from build123d import *

# Parameters (mm, degrees)
F0_W     = 64
F0_H     = 150
F1_DEPTH = 1.5
F2_W     = 48
F2_H     = 39.9
F2_H_2   = 38.8
F2_H_3   = 39.3
F3_DEPTH = 1.501
F4_R     = 8
F6_DEPTH = 4


with BuildPart() as f1:
    # F0 (on Top) → F1 (new body)
    with BuildSketch(Plane.XY):
        with Locations((32, 75)):
            Rectangle(F0_W, F0_H)
    extrude(amount=F1_DEPTH)

    # F2 (on face) → F3 (cut, through all)
    with BuildSketch(Plane.XY.offset(1.5)):
        with Locations((32, 122.05)):
            Rectangle(F2_W, F2_H)
        with Locations((32, 74.7)):
            Rectangle(F2_W, F2_H_2)
        with Locations((32, 27.65)):
            Rectangle(F2_W, F2_H_3)
    extrude(amount=-F3_DEPTH, mode=Mode.SUBTRACT)

    # F4
    f4_edges = [f1.edges().sort_by_distance(p)[0] for p in [
        (8, 142, 0.75),
        (8, 94.1, 0.75),
        (8, 47.3, 0.75),
        (8, 102.1, 0.75),
        (8, 55.3, 0.75),
        (8, 8, 0.75),
        (56, 102.1, 0.75),
        (56, 55.3, 0.75),
        (56, 8, 0.75),
        (56, 142, 0.75),
        (56, 94.1, 0.75),
        (56, 47.3, 0.75),
    ]]
    fillet(f4_edges, radius=F4_R)

    # F5 (on face) → F6 (join)
    with BuildSketch(Plane.XY.offset(1.5)):
        Polygon((0, 0), (64, 0), (64, 0.5), (0.5, 0.5), (0.5, 149.5), (64, 149.5), (64, 150), (0, 150), align=None)
    extrude(amount=F6_DEPTH)


solid = f1.part
Geometry: final body of the model. Coordinates: model frame, mm. A direction names the side the tool comes from. Give positions to 0.01 mm unless a question says otherwise; leave off trailing zeros. Loops run counter-clockwise (first coordinate to the right, second up) from the corner with the lowest first, then second, coordinate; pieces in that order, holes last. Notation, with made-up numbers: (19, -4) - (68, -4) arc R24 ccw to (68, 26) - close; hole circle Ø3 at (19, 22.25). An arc over 180 degrees is marked (long way). Answer as CSV lines item,"result". Start each with the question number.
1. Reachability of faces 1 (the face through (33, 0.5, 3)), 2 (the face through (53.594, 10.281, 0.74)), 3 (the face through (32, 150, 3)) from +Z, -Z, +X, -X, +Y, -Y: full face, straight path, thin tool, end or side. Return the list, or none.
2. Ray query, L1, parallel to Y at x = 24, z = 1.1; L2, parallel to Y at x = 36.5, z = 3.7; L3, parallel to X at y = 34.5, z = 0.85. Return the intervals inside material, ascending.
3. Draft query along X for faces 4 (the face through (53.719, 91.694, 0.74)), 5 (the face through (64, 74.6, 0.5)), 6 (the face through (32, 53, 0)). Return one class per face: released by +X, released by -X, zero draft, split by the parting line, or undercut.
4. Section B-B, the plane y = 67.5. Return loops of the section in (x, z).
5. Section A-A, the plane x = 35. Return loops of the section in (y, z).
6. Section C-C, the plane z = 4. Return loops of the section in (x, y).
7. Section D-D, the plane y = 99. Return loops of the section in (x, z), plus the area to 3 significant figures.
Answers:
1,face 1,"+Z, +X"
1,face 2,"+Z, -Z"
1,face 3,"+Z, -Z, +X, -X, +Y"
2,L1,"y = 0 to 8, 47.3 to 55.3, 94.1 to 102.1, 142 to 150"
2,L2,"y = 0 to 0.5, 149.5 to 150"
2,L3,"x = 0 to 8, 56 to 64"
3,face 4,"undercut"
3,face 5,"released by +X"
3,face 6,"zero draft"
4,outline,"(0, 0) - (8, 0) - (8, 1.5) - (0.5, 1.5) - (0.5, 5.5) - (0, 5.5) - close; (56, 0) - (64, 0) - (64, 1.5) - (56, 1.5) - close"
5,outline,"(0, 0) - (8, 0) - (8, 1.5) - (0.5, 1.5) - (0.5, 5.5) - (0, 5.5) - close; (47.3, 0) - (55.3, 0) - (55.3, 1.5) - (47.3, 1.5) - close; (94.1, 0) - (102.1, 0) - (102.1, 1.5) - (94.1, 1.5) - close; (142, 0) - (150, 0) - (150, 5.5) - (149.5, 5.5) - (149.5, 1.5) - (142, 1.5) - close"
6,outline,"(0, 0) - (64, 0) - (64, 0.5) - (0.5, 0.5) - (0.5, 149.5) - (64, 149.5) - (64, 150) - (0, 150) - close"
7,outline,"(0, 0) - (64, 0) - (64, 1.5) - (0.5, 1.5) - (0.5, 5.5) - (0, 5.5) - close"
7,area,"98.0 mm2"
